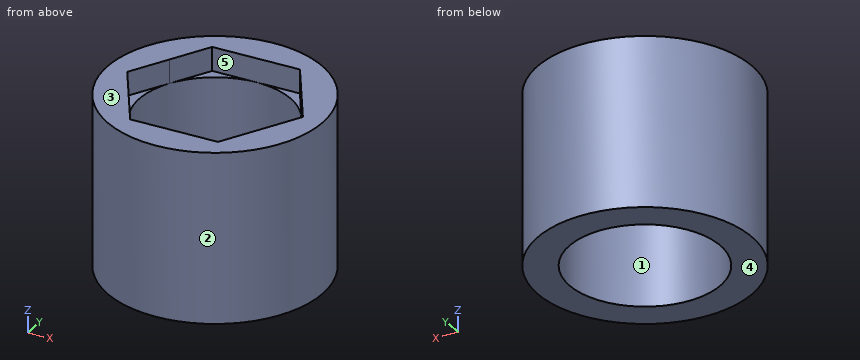
```python
from build123d import *

# Parameters (mm, degrees)
F0_R     = 13.5
F0_R_2   = 9.5
F1_DEPTH = 21.4
F3_DEPTH = 3


with BuildPart() as f1:
    # F0 (on Top) → F1 (new body)
    with BuildSketch(Plane.XY):
        Circle(F0_R)
        Circle(F0_R_2, mode=Mode.SUBTRACT)
    extrude(amount=F1_DEPTH)

    # F2 (on face) → F3 (cut)
    with BuildSketch(Plane.XY.offset(21.4)):
        with BuildLine():
            Line((8.227241, -4.75), (10.969655, 0))
            Line((10.969655, 0), (8.227241, 4.75))
            ThreePointArc((8.227241, 4.75), (9.176295, 2.458781), (9.5, 0))
            ThreePointArc((9.5, 0), (9.176295, -2.458781), (8.227241, -4.75))
        make_face()
        with BuildLine():
            Line((-10.969655, 0), (-8.227241, -4.75))
            ThreePointArc((-8.227241, -4.75), (-9.5, 0), (-8.227241, 4.75))
            Line((-8.227241, 4.75), (-10.969655, 0))
        make_face()
        with BuildLine():
            Line((-5.484828, -9.5), (0, -9.5))
            ThreePointArc((0, -9.5), (-4.75, -8.227241), (-8.227241, -4.75))
            Line((-8.227241, -4.75), (-5.484828, -9.5))
        make_face()
        with BuildLine():
            ThreePointArc((0, 9.5), (4.75, 8.227241), (8.227241, 4.75))
            Line((8.227241, 4.75), (5.484828, 9.5))
            Line((5.484828, 9.5), (0, 9.5))
        make_face()
        with BuildLine():
            Line((5.484828, -9.5), (8.227241, -4.75))
            ThreePointArc((8.227241, -4.75), (4.75, -8.227241), (0, -9.5))
            Line((0, -9.5), (5.484828, -9.5))
        make_face()
        with BuildLine():
            ThreePointArc((-8.227241, 4.75), (-4.75, 8.227241), (0, 9.5))
            Line((0, 9.5), (-5.484828, 9.5))
            Line((-5.484828, 9.5), (-8.227241, 4.75))
        make_face()
    extrude(amount=-F3_DEPTH, mode=Mode.SUBTRACT)


solid = f1.part
```
Geometry: final body of the model. Coordinates: model frame, mm. Face numbers are marked on the shaded views. A direction names the side the tool comes from. Round coordinates to 2 decimals unless told otherwise and drop trailing zeros. Write each loop counter-clockwise with the first axis right and the second up, starting at its lowest first coordinate (ties: lowest second). Pieces come first, ordered by that corner, then holes. Notation, with made-up numbers: (25, 46) -> (48, 46) arc R21 ccw to (48, 68) -> close; hole circle Ø9 at (9.5, 0). An arc over 180 degrees is marked (long way). Use CSV: the item, a comma, the result in double quotes. Start each with the question number.
Q1. Line query: L1, parallel to Y at x = 0, z = 5.5; L2, parallel to Y at x = 4.5, z = 15.5; L3, parallel to X at y = 6.5, z = 13.25. Output: solid intervals per line, ascending.
Q2. Reachability of the marked faces 4 and 5 from +Z, -Z, +X, -X, +Y, -Y: full face, straight path, thin tool, end or side. Return the list, or none.
Q3. First-contact query: pin 1 Ø3.5 at (x, z) = (2.5, 20) entering from -Y; pin 2 Ø5 at (x, y) = (2, 6) entering from +Z; pin 3 Ø12 at (y, z) = (8, 14) entering from -X; pin 4 Ø2.5 at (x, z) = (1.5, 20.5) entering from +Y. Flat tips, straight axial feed; report the tip coordinate or a pass-through.
Q4. Section D-D (x = -10). Return loops of the section in (y, z), plus the area to 3 significant figures.
Q5. Section C-C (z = 3.75). Return loops of the section in (x, y), plus the area to 3 significant figures.
Q6. Section A-A (x = 7.5). Return loops of the section in (y, z).
Q7. Section B-B (y = -2.5). Return loops of the section in (x, z).
Q8. Pull-direction query (Y, two-part tool) for the marked faces 1, 2 and 3; classes: pulls with the +Y half, pulls with the -Y half, needs draft (parallel to the pull), parting line crosses it, or undercut.
Result sheet:
1,L1,"-13.5 to -9.5, 9.5 to 13.5"
1,L2,"-12.73 to -8.37, 8.37 to 12.73"
1,L3,"-11.83 to -6.93, 6.93 to 11.83"
2,face 4,"-Z, +X, -X, +Y, -Y"
2,face 5,"+Z"
3,pin 1,"y = -13.48"
3,pin 2,"through"
3,pin 3,"x = -13.35"
3,pin 4,"y = 13.5"
4,outline,"(-9.07, 0) -> (9.07, 0) -> (9.07, 21.4) -> (1.68, 21.4) -> (1.68, 18.4) -> (-1.68, 18.4) -> (-1.68, 21.4) -> (-9.07, 21.4) -> close"
4,area,"378 mm²"
5,outline,"circle Ø27 at (0, 0); hole circle Ø19 at (0, 0)"
5,area,"289 mm²"
6,outline,"(-11.22, 0) -> (-5.83, 0) -> (-5.83, 18.4) -> (-6.01, 18.4) -> (-6.01, 21.4) -> (-11.22, 21.4) -> close; (5.83, 0) -> (11.22, 0) -> (11.22, 21.4) -> (6.01, 21.4) -> (6.01, 18.4) -> (5.83, 18.4) -> close"
7,outline,"(-13.27, 0) -> (-9.17, 0) -> (-9.17, 18.4) -> (-9.53, 18.4) -> (-9.53, 21.4) -> (-13.27, 21.4) -> close; (9.17, 0) -> (13.27, 0) -> (13.27, 21.4) -> (9.53, 21.4) -> (9.53, 18.4) -> (9.17, 18.4) -> close"
8,face 1,"undercut"
8,face 2,"parting line crosses it"
8,face 3,"needs draft"
